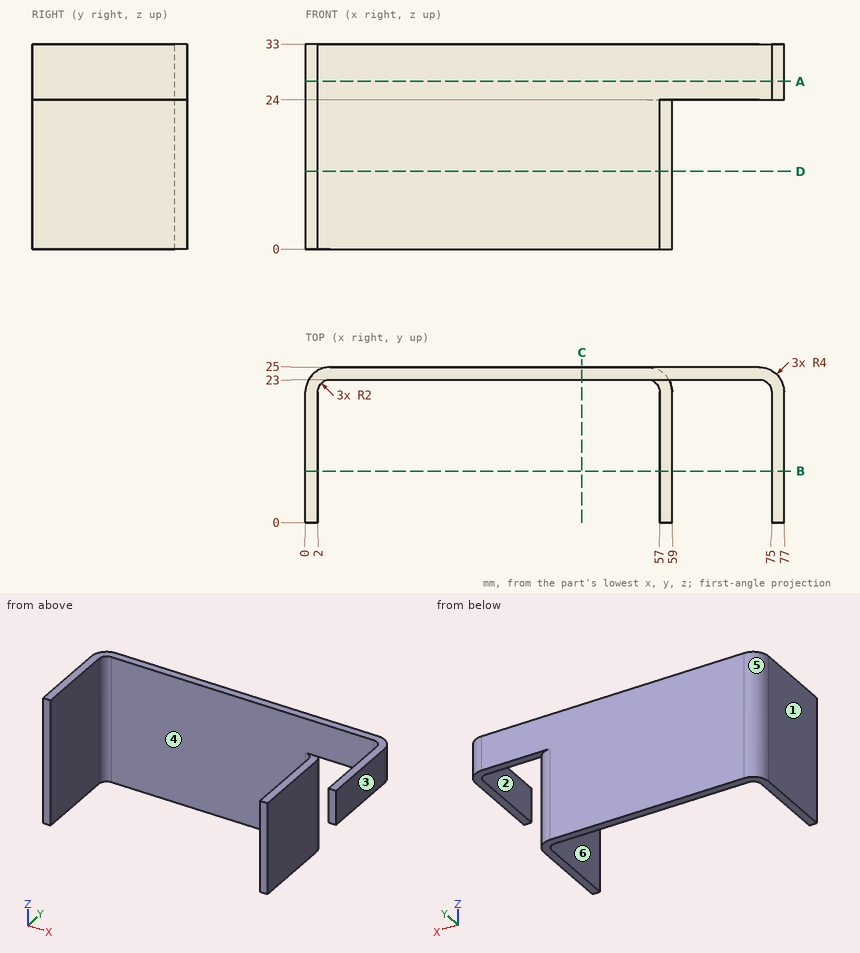
Study the drawing (mm; zero at the part's minimum x, y, z) and answer. A direction names the side the tool comes from. Round coordinates to 2 decimals unless told otherwise and drop trailing zeros. Write each loop counter-clockwise with the first axis right and the second up, starting at its lowest first coordinate (ties: lowest second). Pieces come first, ordered by that corner, then holes.
1) Determine the mould class of the marked faces 1, 2, 3 and 4 for opening direction X: pulls with the +X half, pulls with the -X half, needs draft (parallel to the pull), parting line crosses it, or undercut.
2) Consider probe 1 along X at (y, z) = (19.25, 7.5); probe 2 along X at (y, z) = (8.25, 30); probe 3 along Y at (x, z) = (32, 22). Determine where each line is inside the solid, lowest interval first.
3) Flat-ended cylindrical pins translate along their axes: P1, Ø16.5, axis at x = 36, z = 18.5, coming from the -Y side; P2, Ø12, axis at y = 10.5, z = 12.5, coming from the +X side; P3, Ø1.2, axis at x = 57, y = 15.5, coming from the +Z side; P4, Ø4, axis at x = 62, y = 6.5, coming from the +Z side. Find the tip coordinate at first contact, or state that the pin passes through.
4) Which of the six approach directions +Z, -Z, +X, -X, +Y, -Y give full straight-line access (tool end or side, diameter ignored) to the marked faces 5 and 6?
5) A cutting plane is placed at D-D on z = 12.5. Determine the outline of the cut face in (x, y).
6) A cutting plane is placed at A-A on z = 27. Determine the outline of the cut face in (x, y), and give its area (3 significant figures).
7) A cutting plane is placed at C-C on x = 44.5. Determine the outline of the cut face in (y, z).
8) A cutting plane is placed at B-B on y = 8.25. Determine the outline of the cut face in (x, z), and give its area (3 significant figures).
Entries:
1. face 1: pulls with the -X half
1. face 2: undercut
1. face 3: pulls with the +X half
1. face 4: undercut
2. probe 1: x = 0 to 2, 57 to 59
2. probe 2: x = 0 to 2, 75 to 77
2. probe 3: y = 23 to 25
3. P1: stops at y = 23
3. P2: stops at x = 59
3. P3: stops at z = 24
3. P4: passes through
4. face 5: +Z, -Z, -X, +Y
4. face 6: +Z, -Z, -Y
5. outline: (0, 0) - (2, 0) - (2, 21) arc R2 cw to (4, 23) - (55, 23) arc R2 cw to (57, 21) - (57, 0) - (59, 0) - (59, 21) arc R4 ccw to (55, 25) - (4, 25) arc R4 ccw to (0, 21) - close
6. outline: (0, 0) - (2, 0) - (2, 21) arc R2 cw to (4, 23) - (73, 23) arc R2 cw to (75, 21) - (75, 0) - (77, 0) - (77, 21) arc R4 ccw to (73, 25) - (4, 25) arc R4 ccw to (0, 21) - close
6. area: 241 mm2
7. outline: (23, 0) - (25, 0) - (25, 33) - (23, 33) - close
8. outline: (0, 0) - (2, 0) - (2, 33) - (0, 33) - close; (57, 0) - (59, 0) - (59, 24) - (57, 24) - close; (75, 24) - (77, 24) - (77, 33) - (75, 33) - close
8. area: 132 mm2
